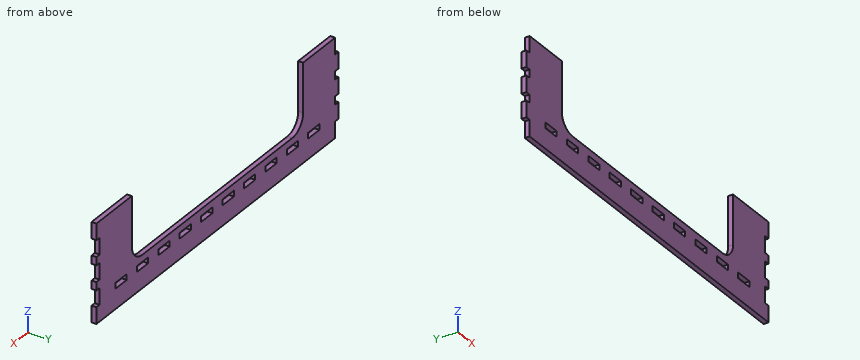
from build123d import *

# Parameters (mm, degrees)
EXTRUDE_1_DEPTH     = 3
SKETCH_2_W          = 10.5
SKETCH_2_H          = 3.5
CUT_EXTRUDE_1_DEPTH = 150.258104234


with BuildPart() as part:
    # Эскиз1 → Бобышка-Вытянуть1 (new body)
    with BuildSketch(Plane(origin=(0, 0, 0), x_dir=(1, 0, 0), z_dir=(0, 1, 0))):
        with BuildLine():
            Line((-135, -31.788922156), (-138, -31.788922156))
            Line((-138, -31.788922156), (-138, -21.788922156))
            Line((-138, -21.788922156), (-135, -21.788922156))
            Line((-135, -21.788922156), (-135, -16.788922156))
            Line((-135, -16.788922156), (-138, -16.788922156))
            Line((-138, -16.788922156), (-138, -6.788922156))
            Line((-138, -6.788922156), (-135, -6.788922156))
            Line((-135, -6.788922156), (-135, 3.211077844))
            Line((-135, 3.211077844), (-125, 3.211077844))
            Line((-125, 3.211077844), (75, 3.211077844))
            Line((75, 3.211077844), (85, 3.211077844))
            Line((85, 3.211077844), (88, 3.211077844))
            Line((88, 3.211077844), (88, -6.788922156))
            Line((88, -6.788922156), (85, -6.788922156))
            Line((85, -6.788922156), (85, -16.788922156))
            Line((85, -16.788922156), (88, -16.788922156))
            Line((88, -16.788922156), (88, -21.788922156))
            Line((88, -21.788922156), (85, -21.788922156))
            Line((85, -21.788922156), (85, -31.788922156))
            Line((85, -31.788922156), (88, -31.788922156))
            Line((88, -31.788922156), (88, -36.788922156))
            Line((88, -36.788922156), (85, -36.788922156))
            Line((85, -36.788922156), (85, -46.788922156))
            Line((85, -46.788922156), (88, -46.788922156))
            Line((88, -46.788922156), (88, -56.788922156))
            Line((88, -56.788922156), (85, -56.788922156))
            Line((85, -56.788922156), (55, -56.788922156))
            Line((55, -56.788922156), (55, -26.788922156))
            ThreePointArc((55, -26.788922156), (52.071067812, -19.717854344), (45, -16.788922156))
            Line((45, -16.788922156), (-95, -16.788922156))
            ThreePointArc((-95, -16.788922156), (-102.071067812, -19.717854344), (-105, -26.788922156))
            Line((-105, -26.788922156), (-105, -56.788922156))
            Line((-105, -56.788922156), (-135, -56.788922156))
            Line((-135, -56.788922156), (-135, -46.788922156))
            Line((-135, -46.788922156), (-138, -46.788922156))
            Line((-138, -46.788922156), (-138, -36.788922156))
            Line((-138, -36.788922156), (-135, -36.788922156))
            Line((-135, -36.788922156), (-135, -31.788922156))
        make_face()
    extrude(amount=EXTRUDE_1_DEPTH)

    # Эскиз2 → Вырез-Вытянуть1 (cut, through all)
    with BuildSketch(Plane(origin=(0, 0, 0), x_dir=(1, 0, 0), z_dir=(0, 1, 0))):
        with Locations((-115, -10.788922156)):
            Rectangle(SKETCH_2_W, SKETCH_2_H)
        with Locations((-95, -10.788922156)):
            Rectangle(SKETCH_2_W, SKETCH_2_H)
        with Locations((-75, -10.788922156)):
            Rectangle(SKETCH_2_W, SKETCH_2_H)
        with Locations((-55, -10.788922156)):
            Rectangle(SKETCH_2_W, SKETCH_2_H)
        with Locations((-35, -10.788922156)):
            Rectangle(SKETCH_2_W, SKETCH_2_H)
        with Locations((-15, -10.788922156)):
            Rectangle(SKETCH_2_W, SKETCH_2_H)
        with Locations((5, -10.788922156)):
            Rectangle(SKETCH_2_W, SKETCH_2_H)
        with Locations((25, -10.788922156)):
            Rectangle(SKETCH_2_W, SKETCH_2_H)
        with Locations((45, -10.788922156)):
            Rectangle(SKETCH_2_W, SKETCH_2_H)
        with Locations((65, -10.788922156)):
            Rectangle(SKETCH_2_W, SKETCH_2_H)
    extrude(amount=CUT_EXTRUDE_1_DEPTH, mode=Mode.SUBTRACT)


solid = part.part
Source: CAD feature listing. Evaluate the final solid. Frame: model axes, mm. Round coordinates to 2 decimals unless told otherwise and drop trailing zeros. Loops run counter-clockwise (first coordinate to the right, second up) from the corner with the lowest first, then second, coordinate; pieces in that order, holes last. Notation, with made-up numbers: (50.25, 89) -> (84.25, 89) arc R28 cw to (84.25, 119) -> close; hole circle Ø5 at (-3.75, 35). An arc over 180 degrees is marked (long way). Answer as a JSON object with one key per item and string values. Group by question number.
Q1. Section query B-B (x = 5). Output: boundary loops of the cut face in (y, z).
Q2. Section query A-A (z = 51). Output: boundary loops of the cut face in (x, y), plus the area to 3 significant figures.
Q3. Contact query for flat-ended pins moving along their axis: P1, Ø1.5, axis at y = 1.5, z = 26, coming from the +X side; P2, Ø1, axis at x = -47.5, y = 0.5, coming from the +Z side. Output: stop coordinate, or through.
Q4. Section query C-C (y = 0.75). State how many separate pieces and enclosed holes the cut face has, plus the area to 3 significant figures.
Q5. Ray query, line 1 (Z direction, x = 61, y = 1.3); line 2 (X direction, y = 1.95, z = 33.5); line 3 (Z direction, x = -12, y = 2.55). Return the intervals inside material, ascending. Write a range as from..to.
Completed:
{
 "1": {"outline": "(0, -3.21) -> (3, -3.21) -> (3, 9.04) -> (0, 9.04) -> close; (0, 12.54) -> (3, 12.54) -> (3, 16.79) -> (0, 16.79) -> close"},
 "2": {"outline": "(-135, 0) -> (-105, 0) -> (-105, 3) -> (-135, 3) -> close; (55, 0) -> (88, 0) -> (88, 3) -> (55, 3) -> close", "area": "189 mm²"},
 "3": {"P1": "x = 85", "P2": "z = 16.79"},
 "4": {"separate pieces": "1", "enclosed holes": "10", "area": "6,660 mm²"},
 "5": {"line 1": "-3.21..9.04, 12.54..56.79", "line 2": "-135..-105, 55..88", "line 3": "-3.21..9.04, 12.54..16.79"}
}
